Study the drawing (mm; zero at the part's minimum x, y, z) and answer. A direction names the side the tool comes from. Coordinates: 2 decimals unless noted, no trailing zeros. Loops run counter-clockwise (first coordinate to the right, second up) from the corner with the lowest first, then second, coordinate; pieces in that order, holes last. Notation, with made-up numbers: (76.25, 13) - (122.25, 13) arc R22 cw to (122.25, 22) - close; hole circle Ø5 at (-4.75, -20.5). An arc over 180 degrees is marked (long way). Put each result on its own line as item: value.
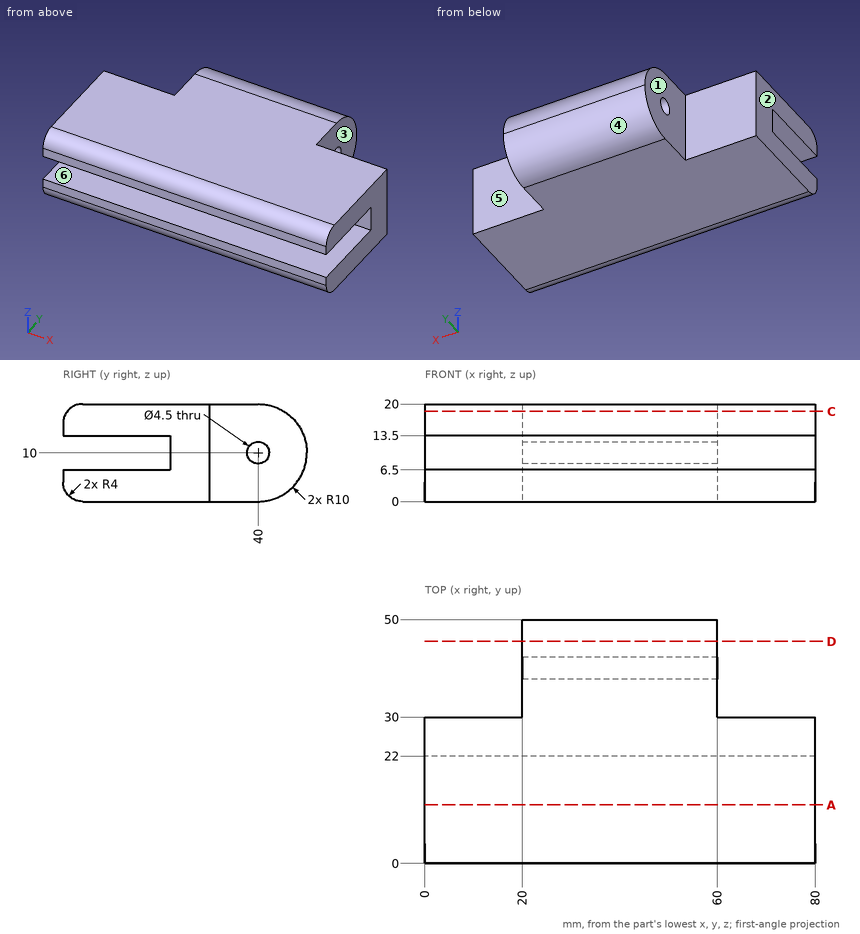
1) Straight lines are drawn through the part: L1, parallel to Y at x = 43, z = 10; L2, parallel to Z at x = 8.5, y = 8.5; L3, parallel to Y at x = 7, z = 7.5. For each, find the intervals that lie inside material, in ascending order. Write a range as [from, to].
Found:
L1: y = [22, 37.75], [42.25, 50]
L2: z = [0, 6.5], [13.5, 20]
L3: y = [22, 30]
2) For the marked faces 1, 2 and 3, determine the directions among +Z, -Z, +X, -X, +Y, -Y from which every point of the face is accessible in a straight line to the end or side of a thin tool.
Found:
face 1: +Z, -Z, -X, +Y
face 2: +Z, -Z, -X, +Y, -Y
face 3: +Z, -Z, +X, +Y
3) The part is cut by section A-A (y = 12). Give the vertices of the cut face in (x, z).
Found:
outline: (0, 0) - (80, 0) - (80, 6.5) - (0, 6.5) - close; (0, 13.5) - (80, 13.5) - (80, 20) - (0, 20) - close
4) Each of these flat-tipped pins is pushed along its axis until it touches: pin 1 (6 mm diameter, centred on y = 40, z = 10, fed in from +X); pin 2 (1.5 mm diameter, centred on x = 35, y = 41, fed in from +Z); pin 3 (1.5 mm diameter, centred on x = 66.5, z = 7.5, fed in from -Y). Where does it stop, or does it pass through?
Found:
pin 1: stops at x = 60
pin 2: stops at z = 20
pin 3: stops at y = 22
5) The part is cut by section C-C (z = 18.5). Give the vertices of the cut face in (x, y).
Found:
outline: (0, 0.88) - (80, 0.88) - (80, 30) - (60, 30) - (60, 45.27) - (20, 45.27) - (20, 30) - (0, 30) - close
6) The part is cut by section D-D (y = 45.5). Give the vertices of the cut face in (x, z).
Found:
outline: (20, 1.65) - (60, 1.65) - (60, 18.35) - (20, 18.35) - close
7) For a pull along Z with two mould halves and no side action, classify the marked faces 4, 5 and 6 as pulls with the +Z half, pulls with the -Z half, needs draft (parallel to the pull), parting line crosses it, or undercut.
Found:
face 4: pulls with the -Z half
face 5: needs draft
face 6: undercut
